```python
from build123d import *

# Parameters (mm, degrees)
BOSS_EXTRUDE1_DEPTH = 10
CUT_EXTRUDE1_DEPTH  = 5
CUT_EXTRUDE2_DEPTH  = 3


with BuildPart() as part:
    # Sketch1 → Boss-Extrude1 (new body)
    with BuildSketch(Plane(origin=(0, 0, 0), x_dir=(1, 0, 0), z_dir=(0, 1, 0))):
        with BuildLine():
            Line((-120, 77.5), (120, 77.5))
            ThreePointArc((120, 77.5), (141.213203436, 68.713203436), (150, 47.5))
            Line((150, 47.5), (150, -47.5))
            ThreePointArc((150, -47.5), (141.213203436, -68.713203436), (120, -77.5))
            Line((120, -77.5), (-120, -77.5))
            ThreePointArc((-120, -77.5), (-141.213203436, -68.713203436), (-150, -47.5))
            Line((-150, -47.5), (-150, 47.5))
            ThreePointArc((-150, 47.5), (-141.213203436, 68.713203436), (-120, 77.5))
        make_face()
    extrude(amount=BOSS_EXTRUDE1_DEPTH)

    # Sketch2 → Cut-Extrude1 (cut)
    with BuildSketch(Plane.XZ):
        with BuildLine():
            Line((-110, 73.5), (110, 73.5))
            ThreePointArc((110, 73.5), (135.455844123, 62.955844123), (146, 37.5))
            Line((146, 37.5), (146, -37.5))
            ThreePointArc((146, -37.5), (135.455844123, -62.955844123), (110, -73.5))
            Line((110, -73.5), (-110, -73.5))
            ThreePointArc((-110, -73.5), (-135.455844123, -62.955844123), (-146, -37.5))
            Line((-146, -37.5), (-146, 37.5))
            ThreePointArc((-146, 37.5), (-135.455844123, 62.955844123), (-110, 73.5))
        make_face()
        with BuildLine():
            Line((-110, 67.5), (110, 67.5))
            ThreePointArc((110, 67.5), (131.213203436, 58.713203436), (140, 37.5))
            Line((140, 37.5), (140, -37.5))
            ThreePointArc((140, -37.5), (131.213203436, -58.713203436), (110, -67.5))
            Line((110, -67.5), (-110, -67.5))
            ThreePointArc((-110, -67.5), (-131.213203436, -58.713203436), (-140, -37.5))
            Line((-140, -37.5), (-140, 37.5))
            ThreePointArc((-140, 37.5), (-131.213203436, 58.713203436), (-110, 67.5))
        make_face(mode=Mode.SUBTRACT)
    extrude(amount=-CUT_EXTRUDE1_DEPTH, mode=Mode.SUBTRACT)

    # Sketch3 → Cut-Extrude2 (cut)
    with BuildSketch(Plane(origin=(0, 10, 0), x_dir=(1, 0, 0), z_dir=(0, 1, 0))):
        with BuildLine():
            Line((-110, 67.5), (110, 67.5))
            ThreePointArc((110, 67.5), (131.213203436, 58.713203436), (140, 37.5))
            Line((140, 37.5), (140, -37.5))
            ThreePointArc((140, -37.5), (131.213203436, -58.713203436), (110, -67.5))
            Line((110, -67.5), (-110, -67.5))
            ThreePointArc((-110, -67.5), (-131.213203436, -58.713203436), (-140, -37.5))
            Line((-140, -37.5), (-140, 37.5))
            ThreePointArc((-140, 37.5), (-131.213203436, 58.713203436), (-110, 67.5))
        make_face()
    extrude(amount=-CUT_EXTRUDE2_DEPTH, mode=Mode.SUBTRACT)


solid = part.part
```
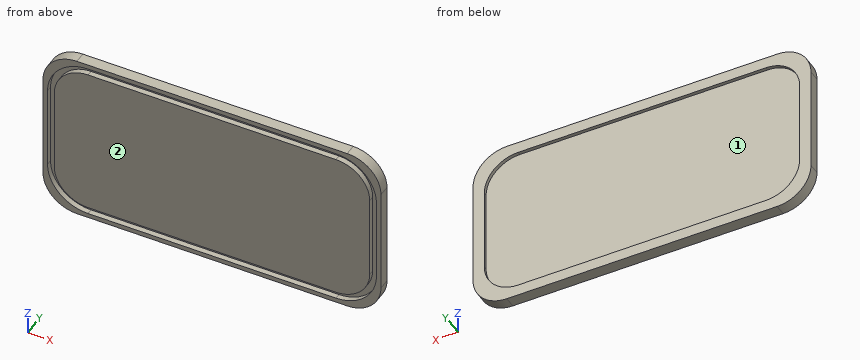
CAD build for the part. Positions are in the model's coordinates, mm. Face numbers are marked on the shaded views. Give positions to 0.01 mm unless a question says otherwise; leave off trailing zeros. Write each loop counter-clockwise with the first axis right and the second up, starting at its lowest first coordinate (ties: lowest second). Pieces come first, ordered by that corner, then holes. Notation, with made-up numbers: M 0,-20 L 40,-20 A10 ccw 40,-5 Z; hole C 28.5,59.25 d8. An arc over 180 degrees is marked long. Return JSON: item names as keys, results as strings. Group by question number.
(1) Band-saw the part on B-B (z = -26). Give the cut face in (x, y).
(2) Band-saw the part on A-A (y = 2). Give the cut face in (x, z).
(3) Mould opens along Z. For the marked faces 1 and 2 say: pulls with the +Z half, pulls with the -Z half, needs draft (parallel to the pull), parting line crosses it, or undercut.
(4) Drill centre lines: L1, parallel to X at y = 0.5, z = -8; L2, parallel to Z at x = -98, y = 2.5; L3, parallel to Z at x = 57.5, y = 8. Where is each one in solid material? Low to high. Write a range as [from, to].
(5) Band-saw the part on C-C (x = -72.5). Give the cut face in (y, z).
(6) Flat gauge pin, fed straight in: pin 1 Ø5 at (y, z) = (8, 55.5) entering from +X. Where does the tip first touch, or does it go through?
Entries:
{
 "1": {"outline": "M -150,0 L -146,0 L -146,5 L -140,5 L -140,0 L 140,0 L 140,5 L 146,5 L 146,0 L 150,0 L 150,10 L 140,10 L 140,7 L -140,7 L -140,10 L -150,10 Z"},
 "2": {"outline": "M -150,-47.5 A30 ccw -120,-77.5 L 120,-77.5 A30 ccw 150,-47.5 L 150,47.5 A30 ccw 120,77.5 L -120,77.5 A30 ccw -150,47.5 Z; M -140,-37.5 A30 ccw -110,-67.5 L 110,-67.5 A30 ccw 140,-37.5 L 140,37.5 A30 ccw 110,67.5 L -110,67.5 A30 ccw -140,37.5 Z; hole M -146,-37.5 A36 ccw -110,-73.5 L 110,-73.5 A36 ccw 146,-37.5 L 146,37.5 A36 ccw 110,73.5 L -110,73.5 A36 ccw -146,37.5 Z"},
 "3": {"face 1": "undercut", "face 2": "needs draft"},
 "4": {"L1": "x = [-150, -146], [-140, 140], [146, 150]", "L2": "z = [-77.5, -73.5], [-67.5, 67.5], [73.5, 77.5]", "L3": "z = [-77.5, -67.5], [67.5, 77.5]"},
 "5": {"outline": "M 0,-77.5 L 10,-77.5 L 10,-67.5 L 7,-67.5 L 7,67.5 L 10,67.5 L 10,77.5 L 0,77.5 L 0,73.5 L 5,73.5 L 5,67.5 L 0,67.5 L 0,-67.5 L 5,-67.5 L 5,-73.5 L 0,-73.5 Z"},
 "6": {"pin 1": "stops at x = 149.49"}
}
